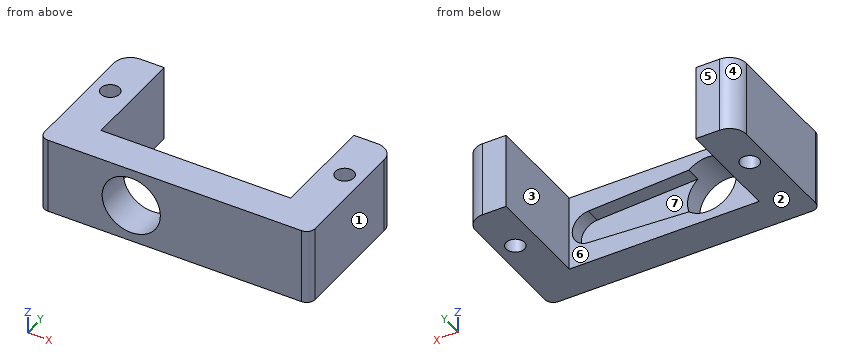
Autodesk Inventor part; units mm, degrees
ref_plane "Work Plane1" through (14.9512, -3.6697, 4.5) normal (-1, 0, 0) x (0, 0, 1)
ref_plane "YZ Plane" through (0, 0, 0) normal (1, 0, 0) x (0, 1, 0)
ref_plane "XZ Plane" through (0, 0, 0) normal (0, 1, 0) x (-1, 0, 0)
sketch "Sketch1" plane through (0, 0, 0) normal (0, 0, 1) x (1, 0, 0)
  line L0 (-1.0988, -7.8697) -> (31.0012, -7.8697)
  line L1 (31.0012, -7.8697) -> (31.0012, 8.8303)
  line L2 (31.0012, 8.8303) -> (26.2012, 8.8303)
  line L3 (26.2012, 8.8303) -> (26.2012, -3.6697)
  line L4 (26.2012, -3.6697) -> (3.7012, -3.6697)
  line L5 (3.7012, -3.6697) -> (3.7012, 8.8303)
  line L6 (3.7012, 8.8303) -> (-1.0988, 8.8303)
  line L7 (-1.0988, 8.8303) -> (-1.0988, -7.8697)
  dimension "d5" = 4.8
  dimension "d6" = 22.5
  dimension "d7" = 12.5
  dimension "d8" = 4.2
extrude "Extrusion1" add sketch "Sketch1" along normal mid plane 9
sketch "Sketch2" plane through (0, 0, 4.5) normal (0, 0, 1) x (1, 0, 0)
  line L0 (3.7012, -3.6697) -> (3.7012, 8.8303)
  line L1 (3.7012, 8.8303) -> (-1.0988, 8.8303)
  point P0 (0, 0)
  point P1 (3.7012, 2.5803)
  point P2 (3.7012, 2.5803)
  point P3 (1.0512, 2.5803)
  point P4 (3.7012, 2.5803)
  point P5 (3.7012, 2.5803)
  dimension "d14" = 2.65
hole "Hole1" at (1.0512, 2.5803, 4.5) direction (0, 0, -1) diameter 2.2 end through all
ref_plane "Work Plane1" through (14.9512, -3.6697, 4.5) normal (-1, 0, 0) x (0, 0, 1)
mirror "Mirror1" about plane through (14.9512, -3.6697, 4.5) normal (-1, 0, 0) of "Hole1"
sketch "Sketch4" plane through (3.7012, -3.6697, 4.5) normal (0, 1, 0) x (1, 0, 0)
  line L0 (0, 9) -> (0, 0)
  line L1 (22.5, 0) -> (0, 0)
  line L2 (22.5, 9) -> (22.5, 0)
  line L3 (0, 9) -> (22.5, 9)
  circle A0 centre (6.1, 4.5) radius 3.45
  line L4 (8.3091, 7.15) -> (8.3091, 1.85) construction
  arc A1 (20.2591, 2.503) -> (20.2591, 6.497) centre (20.15, 4.5) ccw
  line L5 (8.3091, 7.15) -> (20.2591, 6.497)
  line L6 (8.3091, 1.85) -> (20.2591, 2.503)
  line L7 (6.1, 4.5) -> (20.15, 4.5) construction
  line L8 (0, 9) -> (0, 0)
  line L9 (0, 9) -> (0, 0)
  point P0 (-3.7012, 4.5)
  point P1 (11.25, 9)
  point P2 (0, 4.5)
  point P3 (0, 4.5)
  dimension "d23" = 5.3
  dimension "d25" = 2
  dimension "d26" = 14.05
  dimension "d27" = 6.9
  dimension "d28" = 6.1
extrude "Extrusion2" cut sketch "Sketch4" against normal through all contours A0
extrude "Extrusion3" cut sketch "Sketch4" against normal blind 1.8 contours A0 L5 A1 L6
fillet "Fillet1" radius 2 2 edges at (-1.0988, 8.8303, 0) (31.0012, 8.8303, 0)
fillet "Fillet1" radius 1 2 edges at (31.0012, -7.8697, 0) (-1.0988, -7.8697, 0)
properties part number "Hip v0.1"
Geometry: final body of the model. Coordinates: model frame, mm. Face numbers are marked on the shaded views. A direction names the side the tool comes from. Give positions to 0.01 mm unless a question says otherwise; leave off trailing zeros. Loops run counter-clockwise (first coordinate to the right, second up) from the corner with the lowest first, then second, coordinate; pieces in that order, holes last. Notation, with made-up numbers: M 36,1.5 L 48,1.5 A16 ccw 48,9.5 Z; hole C 70,-12 d10. An arc over 180 degrees is marked long. Put each result on its own line as item: value. Start each with the question number.
1) Cut plane D-D (y = 2.75). Output: boundary loops of the cut face in (x, z), then the cut area to 3 significant figures.
2) Cut plane B-B (x = 10). Output: boundary loops of the cut face in (y, z), then the cut area to 3 significant figures.
3) Ray query, line 1 along Z through (x, y) = (12, -7); line 2 along X through (y, z) = (4.25, -0.25); line 3 along Z through (x, y) = (10, -5.75). Return the intervals inside material, ascending.
4) Cut plane A-A (y = -2). Output: boundary loops of the cut face in (x, z).
5) Pull-direction query (X, two-part tool) for the marked faces 1, 2, 3 and 4; classes: pulls with the +X half, pulls with the -X half, needs draft (parallel to the pull), parting line crosses it, or undercut.
6) Contact query for flat-ended pins moving along their axis: pin 1 (1.8 mm diameter, centred on x = 28.85, y = 2.58, fed in from -Z); pin 2 (4 mm diameter, centred on x = 15.5, z = 0.5, fed in from +Y); pin 3 (3 mm diameter, centred on x = 17.5, z = -0.5, fed in from +Y). Output: stop coordinate, or through.
7) Cut plane C-C (z = 0.5). Output: boundary loops of the cut face in (x, y), then the cut area to 3 significant figures.
8) Access query for the marked faces 5, 6 and 7. Directions: +Z, -Z, +X, -X, +Y, -Y. A direction counts if a zero-diameter tool reaches every point of the face in a straight line with its end or side. Return the directions, or none.
Verdict:
1. outline: M -1.1,-4.5 L -0.04,-4.5 L -0.04,4.5 L -1.1,4.5 Z; M 2.14,-4.5 L 3.7,-4.5 L 3.7,4.5 L 2.14,4.5 Z; M 26.2,-4.5 L 27.76,-4.5 L 27.76,4.5 L 26.2,4.5 Z; M 29.94,-4.5 L 31,-4.5 L 31,4.5 L 29.94,4.5 Z
1. area: 47.3 mm2
2. outline: M -7.87,-4.5 L -3.67,-4.5 L -3.67,-3.44 L -7.87,-3.44 Z; M -7.87,3.44 L -3.67,3.44 L -3.67,4.5 L -7.87,4.5 Z
2. area: 8.87 mm2
3. line 1: -4.5 to -2.66, 2.66 to 4.5
3. line 2: -1.1 to 3.7, 26.2 to 31
3. line 3: -4.5 to -3.44, 3.44 to 4.5
4. outline: M -1.1,-4.5 L 3.7,-4.5 L 3.7,4.5 L -1.1,4.5 Z; M 26.2,-4.5 L 31,-4.5 L 31,4.5 L 26.2,4.5 Z
5. face 1: pulls with the +X half
5. face 2: needs draft
5. face 3: undercut
5. face 4: pulls with the -X half
6. pin 1: through
6. pin 2: y = -3.67
6. pin 3: y = -5.47
7. outline: M -1.1,-6.87 A1 ccw -0.1,-7.87 L 6.39,-7.87 L 6.39,-3.67 L 3.7,-3.67 L 3.7,8.83 L 0.9,8.83 A2 ccw -1.1,6.83 Z; M 13.21,-7.87 L 30,-7.87 A1 ccw 31,-6.87 L 31,6.83 A2 ccw 29,8.83 L 26.2,8.83 L 26.2,-3.67 L 25.79,-3.67 L 25.79,-5.47 L 13.21,-5.47 Z; hole C 1.05,2.58 d2.2; hole C 28.85,2.58 d2.2
7. area: 194 mm2
8. face 5: +Z, -Z, +X, -X, +Y
8. face 6: +Z, -Z, +Y
8. face 7: +Y
